```python
from build123d import *

# Parameters (mm, degrees)
SKETCH086_W     = 44
SKETCH086_H     = 20
PAD047_DEPTH    = 99
SKETCH087_W     = 39.5
SKETCH087_H     = 11.5
PAD048_DEPTH    = 30.5
SKETCH088_W     = 30
SKETCH088_H     = 7
POCKET031_DEPTH = 129.5
SKETCH089_W     = 40
SKETCH089_H     = 12
POCKET032_DEPTH = 31
CHAMFER051_SIZE = 0.5
CHAMFER052_SIZE = 0.5
CHAMFER053_SIZE = 0.5


with BuildPart() as part:
    # Sketch086 → Pad047 (new body)
    with BuildSketch(Plane.YZ):
        Rectangle(SKETCH086_W, SKETCH086_H)
    extrude(amount=PAD047_DEPTH)

    # Sketch087 (on Face5 of Pad047) → Pad048 (join)
    with BuildSketch(Plane(origin=(0, 0, 0), x_dir=(0, 1, 0), z_dir=(-1, 0, 0))):
        Rectangle(SKETCH087_W, SKETCH087_H)
    extrude(amount=PAD048_DEPTH)

    # Sketch088 (on Face5 of Pad048) → Pocket031 (cut)
    with BuildSketch(Plane.YZ.offset(99)):
        Rectangle(SKETCH088_W, SKETCH088_H)
    extrude(amount=-POCKET031_DEPTH, mode=Mode.SUBTRACT)

    # Sketch089 (on Face5 of Pocket031) → Pocket032 (cut)
    with BuildSketch(Plane.YZ.offset(99)):
        Rectangle(SKETCH089_W, SKETCH089_H)
    extrude(amount=-POCKET032_DEPTH, mode=Mode.SUBTRACT)

    # Chamfer051
    chamfer051_edges = [part.edges().sort_by_distance(p)[0] for p in [
        (-30.5, 0, -5.75),
        (-30.5, -19.75, 0),
        (-30.5, 19.75, 0),
        (-30.5, 0, 5.75),
        (-30.5, -15, 0),
        (-30.5, 0, -3.5),
        (-30.5, 15, 0),
        (-30.5, 0, 3.5),
        (-15.25, 19.75, 5.75),
        (-15.25, -19.75, 5.75),
        (-15.25, 19.75, -5.75),
        (-15.25, -19.75, -5.75),
    ]]
    chamfer(chamfer051_edges, length=CHAMFER051_SIZE)

    # Chamfer052
    chamfer052_edges = [part.edges().sort_by_distance(p)[0] for p in [
        (99, 0, 6),
        (99, -20, 0),
        (99, 0, -6),
        (99, 20, 0),
    ]]
    chamfer(chamfer052_edges, length=CHAMFER052_SIZE)

    # Chamfer053
    chamfer053_edges = [part.edges().sort_by_distance(p)[0] for p in [
        (49.5, -22, 10),
        (49.5, -22, -10),
        (49.5, 22, 10),
        (49.5, 22, -10),
    ]]
    chamfer(chamfer053_edges, length=CHAMFER053_SIZE)


with BuildPart() as part_1:
    # Body016 placement: moved
    add(part.part.moved(Location((0, 75, 4))))


solid = part_1.part
```
Verification items for the finished model (mm, model axes). A direction names the side the tool comes from. Coordinates: 2 decimals unless noted, no trailing zeros. Loops run counter-clockwise (first coordinate to the right, second up) from the corner with the lowest first, then second, coordinate; pieces in that order, holes last. Notation, with made-up numbers: (-22.5, -39.5) -> (-18.5, -39.5) arc R38 ccw to (-18.5, -0.5) -> close; hole circle Ø4 at (22.25, 21.25). An arc over 180 degrees is marked (long way). Answer in a Markdown table with one row per item. Add a question column.
1. Section check D-D, the plane y = 92.5. Enter the section's corners in (x, z).
2. Access from +Z, -Z, +X, -X, +Y, -Y to the whole of each face (thin tool, end or side, straight path). Record for faces 4 (the face through (68, 75, 8)), 5 (the face through (-15, 55.25, 4)), 6 (the face through (-15, 94.75, 4)), 7 (the face through (20, 75, 7.5)), 8 (the face through (-15, 75, -1.75)).
3. Depth check by flat-ended pin: P1, Ø3, axis at x = -19.5, z = 4, coming from the +Y side; P2, Ø3, axis at x = -13.5, z = 3.5, coming from the -Y side; P3, Ø6, axis at x = -0.5, y = 60, coming from the +Z side; P4, Ø5, axis at x = -5.5, y = 64, coming from the +Z side. Enter the tip coordinate at first touch or a pass-through.
4. Material ranges on probe 1 along Z at (x, y) = (36, 74.5); probe 2 along Y at (x, z) = (84, 9); probe 3 along Y at (x, z) = (-13, 2), recorded low to high. Write a range as [from, to].
5. Draft check along Z on faces 1 (the face through (49, 53, 4)), 2 (the face through (-15, 75, 9.75)), 3 (the face through (83, 75, -2)). Enter one of: +Z half, -Z half, draft (parallel to the pull), parting line (faces both ways), or undercut.
6. Section check B-B, the plane z = 6. Enter the section's corners in (x, y).
7. Section check C-C, the plane x = 31.5. Enter the section's corners in (y, z).
8. Section check A-A, the plane y = 69. Enter the section's corners in (x, z), then the cut area to 3 significant figures.
Derived:
| question | item | result |
|---|---|---|
| 1 | outline | (-30.5, -1.25) -> (-30, -1.75) -> (0, -1.75) -> (0, -6) -> (99, -6) -> (99, -2.5) -> (98.5, -2) -> (68, -2) -> (68, 10) -> (98.5, 10) -> (99, 10.5) -> (99, 14) -> (0, 14) -> (0, 9.75) -> (-30, 9.75) -> (-30.5, 9.25) -> close |
| 2 | face 4 | +X |
| 2 | face 5 | +Z, -Z, -X, -Y |
| 2 | face 6 | +Z, -Z, -X, +Y |
| 2 | face 7 | +X, -X |
| 2 | face 8 | -Z, -X, +Y, -Y |
| 3 | P1 | stops at y = 94.75 |
| 3 | P2 | stops at y = 55.25 |
| 3 | P3 | stops at z = 14 |
| 3 | P4 | stops at z = 9.75 |
| 4 | probe 1 | z = [-6, 0.5], [7.5, 14] |
| 4 | probe 2 | y = [53, 55], [95, 97] |
| 4 | probe 3 | y = [55.25, 60], [90, 94.75] |
| 5 | face 1 | draft |
| 5 | face 2 | +Z half |
| 5 | face 3 | undercut |
| 6 | outline | (-30.5, 55.75) -> (-30, 55.25) -> (0, 55.25) -> (0, 53) -> (99, 53) -> (99, 54.5) -> (98.5, 55) -> (68, 55) -> (68, 60) -> (-30, 60) -> (-30.5, 59.5) -> close; (-30.5, 90.5) -> (-30, 90) -> (68, 90) -> (68, 95) -> (98.5, 95) -> (99, 95.5) -> (99, 97) -> (0, 97) -> (0, 94.75) -> (-30, 94.75) -> (-30.5, 94.25) -> close |
| 7 | outline | (53, -5.5) -> (53.5, -6) -> (96.5, -6) -> (97, -5.5) -> (97, 13.5) -> (96.5, 14) -> (53.5, 14) -> (53, 13.5) -> close; hole (60, 0.5) -> (90, 0.5) -> (90, 7.5) -> (60, 7.5) -> close |
| 8 | outline | (-30.5, -1.25) -> (-30, -1.75) -> (0, -1.75) -> (0, -6) -> (99, -6) -> (99, -2.5) -> (98.5, -2) -> (68, -2) -> (68, 0.5) -> (-30, 0.5) -> (-30.5, 0) -> close; (-30.5, 8) -> (-30, 7.5) -> (68, 7.5) -> (68, 10) -> (98.5, 10) -> (99, 10.5) -> (99, 14) -> (0, 14) -> (0, 9.75) -> (-30, 9.75) -> (-30.5, 9.25) -> close |
| 8 | area | 1,270 mm² |
